Here's how the part is built. I have some questions about the finished solid (model axes, mm). Face numbers are marked on the shaded views. A direction names the side the tool comes from. Round coordinates to 2 decimals unless told otherwise and drop trailing zeros. Write each loop counter-clockwise with the first axis right and the second up, starting at its lowest first coordinate (ties: lowest second). Pieces come first, ordered by that corner, then holes. Notation, with made-up numbers: (33.5, 0.25) - (60.5, 0.25) arc R27 cw to (60.5, 26.25) - close; hole circle Ø7 at (77.5, -35.75). An arc over 180 degrees is marked (long way). Write item = value, one per line. Start each with the question number.
Item 1: If we section it at D-D (x = 69): Please give me the cut outline in (y, z).
Item 2: If we section it at C-C (z = -42.5): Please give me the cut outline in (x, y), and give its area (3 significant figures).
Item 3: For P1, Ø10, axis at y = 124, z = -20.5, coming from the +X side; P2, Ø8, axis at y = 130.5, z = -6.5, coming from the +X side; P3, Ø10, axis at x = 20.5, y = 54.5, coming from the -Z side, each with a flat end and sliding along its axis, tell me the tip position at first contact or that it passes through.
Item 4: Thinking about a two-plate mould opening in X: for the marked faces 3, 4 and 5, which applies, pulls with the +X half, pulls with the -X half, needs draft (parallel to the pull), parting line crosses it, or undercut?
Item 5: If I drill on line 1 along Y through (x, z) = (51.5, -25.5); line 2 along Z through (x, y) = (11, 182); line 3 along X through (y, z) = (248, -11), over which ranges is the centre line in solid material (lowest first)? Write a range as [from, to].
Item 6: Which directions (+Z, -Z, +X, -X, +Y, -Y) give clear straight access to the entire face, cutting with the end or side of a thin tool? Please do the marked faces 1 and 2.
Item 7: If we section it at B-B (x = -28): Please give me the cut outline in (y, z), and give its area (3 significant figures).
Item 8: If we section it at A-A (z = -56.5): Please give me the cut outline in (x, y).
```python
from build123d import *

# Parameters (mm, degrees)
BOSS_EXTRUDE1_DEPTH = 260
CUT_EXTRUDE1_DEPTH  = 256


with BuildPart() as part:
    # Sketch1 → Boss-Extrude1 (new body)
    with BuildSketch(Plane(origin=(0, 0, 0), x_dir=(1, 0, 0), z_dir=(0, 1, 0))):
        with BuildLine():
            Line((35, 0), (-35, 0))
            ThreePointArc((-35, 0), (-52.207293091, 5.425438671), (-63.190778624, 19.7393957))
            Line((-63.190778624, 19.7393957), (-81.908713693, 64.7393957))
            Line((-81.908713693, 64.7393957), (81.908713693, 64.7393957))
            Line((81.908713693, 64.7393957), (63.190778624, 19.7393957))
            ThreePointArc((63.190778624, 19.7393957), (52.207293091, 5.425438671), (35, 0))
        make_face()
    extrude(amount=BOSS_EXTRUDE1_DEPTH)

    # Sketch4 → Cut-Extrude1 (cut)
    with BuildSketch(Plane.XZ):
        with BuildLine():
            Line((-78.908713693, -64.7393957), (78.908713693, -64.7393957))
            Line((78.908713693, -64.7393957), (60.788869437, -21.764400459))
            add(Edge.make_bspline(
                [(35, -3), (54.769523096, -6.842262635), (60.788869437, -21.764400459)],
                knots=[0, 0, 0, 1, 1, 1], degree=2))
            Line((35, -3), (-35, -3))
            add(Edge.make_bspline(
                [(-35, -3), (-54.769523096, -6.842262635), (-60.788869437, -21.764400459)],
                knots=[0, 0, 0, 1, 1, 1], degree=2))
            Line((-60.788869437, -21.764400459), (-78.908713693, -64.7393957))
        make_face()
    extrude(amount=-CUT_EXTRUDE1_DEPTH, mode=Mode.SUBTRACT)


solid = part.part
```
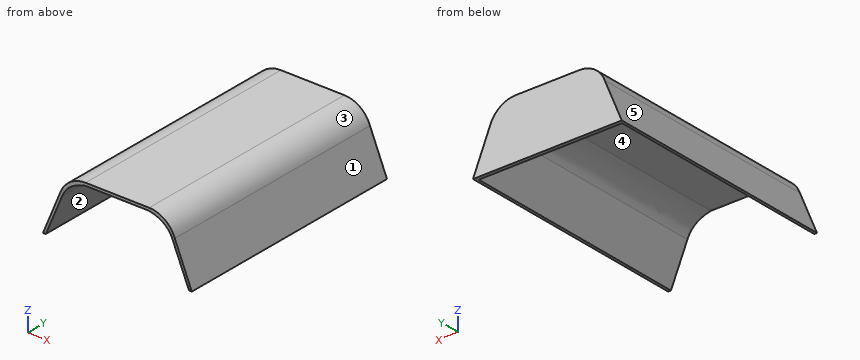
Reply:
q1.outline = (0, -41.24) - (256, -41.24) - (256, -64.74) - (260, -64.74) - (260, -33.71) - (0, -33.71) - close
q2.outline = (-72.66, 0) - (-69.53, 0) - (-69.53, 256) - (69.53, 256) - (69.53, 0) - (72.66, 0) - (72.66, 260) - (-72.66, 260) - close
q2.area = 2,180 mm2
q3.P1 = 65.59
q3.P2 = 57.8
q3.P3 = -3
q4.face_3 = pulls with the +X half
q4.face_4 = undercut
q4.face_5 = pulls with the -X half
q5.line_1 = [256, 260]
q5.line_2 = [-3, 0]
q5.line_3 = [-58.22, -53.09], [53.09, 58.22]
q6.face_1 = +Z, +X, +Y, -Y
q6.face_2 = -Z, -Y
q7.outline = (0, -3) - (256, -3) - (256, -64.74) - (260, -64.74) - (260, 0) - (0, 0) - close
q7.area = 1,030 mm2
q8.outline = (-78.48, 0) - (-75.43, 0) - (-75.43, 256) - (75.43, 256) - (75.43, 0) - (78.48, 0) - (78.48, 260) - (-78.48, 260) - close
